Source: CAD feature listing. Evaluate the final solid. Frame: model axes, mm. A direction names the side the tool comes from. Give positions to 0.01 mm unless a question says otherwise; leave off trailing zeros. Write each loop counter-clockwise with the first axis right and the second up, starting at its lowest first coordinate (ties: lowest second). Pieces come first, ordered by that corner, then holes. Notation, with made-up numbers: (-24.5, 63) -> (20.5, 63) arc R15 ccw to (20.5, 71) -> close; hole circle Ø9 at (35, -16.5). An arc over 180 degrees is marked (long way). Answer as a JSON object with one key per item and string values. Group by question number.
Item 1: Section query D-D on x = 0. Return the cut outline in (y, z), plus the area to 3 significant figures.
Item 2: Section query A-A on z = 0. Return the cut outline in (x, y), plus the area to 3 significant figures.
Item 3: Section query B-B on x = 4.25. Return the cut outline in (y, z).
Item 4: Section query C-C on y = 3.9. Return the cut outline in (x, z).
Item 5: First-contact query: pin 1 Ø0.6 at (y, z) = (4, -8.5) entering from +X; pin 2 Ø1.5 at (x, y) = (4.5, 1) entering from +Z; pin 3 Ø1.5 at (y, z) = (3, 6) entering from -X. Flat tips, straight axial feed; report the tip coordinate or a pass-through.
Item 6: Ray query, probe 1 along Y at (x, z) = (-5, 7.75); probe 2 along X at (y, z) = (1.55, 7.75); probe 3 along Z at (x, y) = (4.75, 2). Return the intervals inside material, ascending. Write a range as from..to.
Item 7: Access query for faces 1 (the face through (0.265, 4.006, 6.495)), 2 (the face through (1.5, 4, -8)), 3 (the face through (-1.5, 4, -8)). Directions: +Z, -Z, +X, -X, +Y, -Y. A direction counts if a zero-diameter tool reaches every point of the face in a straight line with its end or side. Return the directions, or none.
from build123d import *

# Parameters (mm, degrees)
BOSS_EXTRUDE1_DEPTH = 0.8


with BuildPart() as part:
    # Sketch1 → Revolve1 (revolve)
    with BuildSketch(Plane(origin=(0, 0, 0), x_dir=(0, 0, -1), z_dir=(1, 0, 0))):
        Polygon((0, 0), (9.9, 0), (9.9, 3.6), (6.5, 3.6), (6.5, 4.4), (0, 4.4), align=None)
    revolve(axis=Axis((0, 4.4, 0), (0, -1, 0)))

    # Sketch2 → Boss-Extrude1 (add)
    with BuildSketch(Plane(origin=(0, 3.6, 0), x_dir=(1, 0, 0), z_dir=(0, 1, 0))):
        with BuildLine():
            Line((-1.5, 6.32455532), (1.5, 6.32455532))
            Line((1.5, 6.32455532), (1.5, 9.785703858))
            ThreePointArc((1.5, 9.785703858), (0, 9.9), (-1.5, 9.785703858))
            Line((-1.5, 9.785703858), (-1.5, 6.32455532))
        make_face()
    extrude(amount=BOSS_EXTRUDE1_DEPTH)


solid = part.part
Worked answers:
{
 "1": {"outline": "(0, -9.9) -> (4.4, -9.9) -> (4.4, 6.5) -> (3.6, 6.5) -> (3.6, 9.9) -> (0, 9.9) -> close", "area": "84.4 mm^2"},
 "2": {"outline": "(-9.9, 0) -> (9.9, 0) -> (9.9, 3.6) -> (6.5, 3.6) -> (6.5, 4.4) -> (-6.5, 4.4) -> (-6.5, 3.6) -> (-9.9, 3.6) -> close", "area": "81.7 mm^2"},
 "3": {"outline": "(0, -8.94) -> (3.6, -8.94) -> (3.6, -4.92) -> (4.4, -4.92) -> (4.4, 4.92) -> (3.6, 4.92) -> (3.6, 8.94) -> (0, 8.94) -> close"},
 "4": {"outline": "(-1.5, -9.79) arc R9.9 ccw to (1.5, -9.79) -> (1.5, -6.32) arc R6.5 ccw (long way) to (-1.5, -6.32) -> close"},
 "5": {"pin 1": "x = 1.5", "pin 2": "z = 9.16", "pin 3": "x = -8.39"},
 "6": {"probe 1": "0..3.6", "probe 2": "-6.16..6.16", "probe 3": "-8.69..8.69"},
 "7": {"face 1": "+Y", "face 2": "-Z, +X, +Y", "face 3": "-Z, -X, +Y"}
}
